CAD build for the part. Positions are in the model's coordinates, mm. Face numbers are marked on the shaded views. A direction names the side the tool comes from. Coordinates: 2 decimals unless noted, no trailing zeros. Order: outer loops, then holes, each group sorted by start corner. A loop starts at its lowest first (then second) coordinate and runs counter-clockwise, first axis right, second up. Notation, with made-up numbers: (-7, 6.5) - (22, 6.5) arc R30 cw to (22, 28.5) - close; hole circle Ø10 at (39, 6). An arc over 180 degrees is marked (long way). Use one line per item in the form item = value.
```python
from build123d import *

# Parameters (mm, degrees)
F0_W     = 800
F0_H     = 400
F1_DEPTH = 150
F2_R     = 94.1543289326
F3_T     = -30
F4_DEPTH = 202


with BuildPart() as f1:
    # F0 (on Top) → F1 (new body)
    with BuildSketch(Plane.XY):
        Rectangle(F0_W, F0_H)
    extrude(amount=F1_DEPTH)

    # F2
    f2_edges = [f1.edges().sort_by_distance(p)[0] for p in [
        (-400, 200, 75),
        (-400, -200, 75),
    ]]
    fillet(f2_edges, radius=F2_R)

    # F3
    f3_openings = [f1.faces().sort_by_distance(p)[0] for p in [
        (4.56029, 0, 150),
    ]]
    offset(amount=F3_T, openings=f3_openings)

    # F4 (cut): a face of the model
    f4_faces = [f1.faces().sort_by_distance(p)[0] for p in [
        (2.5148489981, 0, 30),
    ]]
    extrude(f4_faces, amount=-F4_DEPTH, mode=Mode.SUBTRACT)


solid = f1.part
```
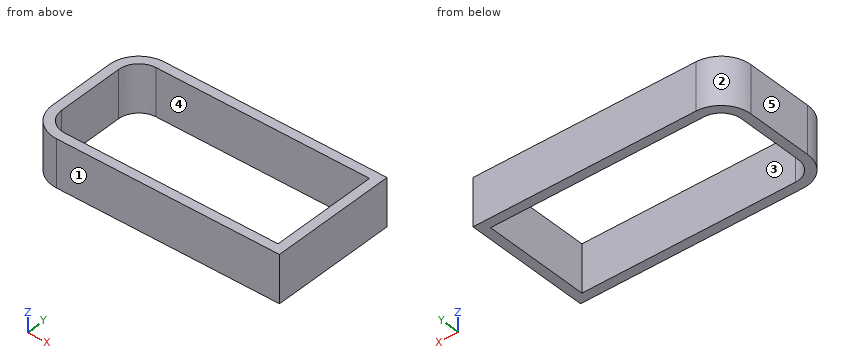
Item 1: Drill centre lines: line 1 (X direction, y = -81.5, z = 70.5); line 2 (Y direction, x = -237.5, z = 99.5); line 3 (X direction, y = -109.5, z = 51.5). Where is each one in solid material? Low to high. Write a range as [from, to].
Derived:
line_1 = [-400, -370], [370, 400]
line_2 = [-200, -170], [170, 200]
line_3 = [-399.93, -369.9], [370, 400]
Item 2: Drop a flat-ended pin along its axis: pin 1 (5 mm diameter, centred on y = -156, z = 132.5, fed in from -X). Give the stop position or say it passes through.
Derived:
pin_1 = -387.05
Item 3: 3-axis set-ups, long thin cutter, end or side, ignore diameter. For the marked faces 4 and 5: which of +Z, -Z, +X, -X, +Y, -Y reach the whole face in a straight line?
Derived:
face_4 = +Z, -Z
face_5 = +Z, -Z, -X, +Y, -Y
Item 4: Two-plate mould, pull along Y, no slides. Class the marked faces 1, 2 and 3: +Y half, -Y half, draft (parallel to the pull), parting line (faces both ways), or undercut.
Derived:
face_1 = -Y half
face_2 = +Y half
face_3 = undercut
Item 5: Cut at A-A, the plane y = 77. Write the cut outline in (x, z), plus the area to 3 significant figures.
Derived:
outline = (-400, 0) - (-370, 0) - (-370, 150) - (-400, 150) - close; (370, 0) - (400, 0) - (400, 150) - (370, 150) - close
area = 9,000 mm²
Item 6: Cut at B-B, the plane x = 295.5. Write the cut outline in (y, z).
Derived:
outline = (-200, 0) - (-170, 0) - (-170, 150) - (-200, 150) - close; (170, 0) - (200, 0) - (200, 150) - (170, 150) - close
Item 7: Cut at C-C, the plane z = 115.5. Write the cut outline in (x, y), plus the area to 3 significant figures.
Derived:
outline = (-400, -105.85) arc R94.15 ccw to (-305.85, -200) - (400, -200) - (400, 200) - (-305.85, 200) arc R94.15 ccw to (-400, 105.85) - close; hole (-370, -105.85) arc R64.15 ccw to (-305.85, -170) - (370, -170) - (370, 170) - (-305.85, 170) arc R64.15 ccw to (-370, 105.85) - close
area = 66,400 mm²
